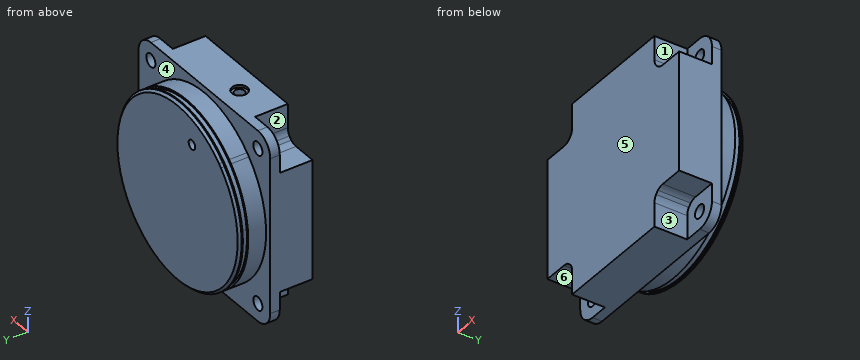
from build123d import *

# Parameters (mm, degrees)
F1_DEPTH        = 58
F0_R            = 5.5
F2_DEPTH        = 35.5
F3_DEPTH        = 35.5
F3_COPIES_COUNT = 4
F4_DEPTH        = 27.5
F4_COPIES_COUNT = 4
F5_SIZE         = 2
F7_D            = 8.5
F7_DEPTH        = 35
F7_CBORE_D      = 13
F7_CBORE_DEPTH  = 2
F7_TIP          = 2.5536576309
F9_D            = 8
F9_DEPTH        = 40
F9_TIP          = 2.4034424761
F10_W           = 4.5
F10_H           = 1.5


# Not quite as in the source:
# - a pattern or mirror of a feature is missing from the dataset's text; its kind, count and spacing are read off the source's solid


with BuildPart() as f1:
    # F0 (on Front) → F1 (new body)
    with BuildSketch(Plane.XZ):
        with BuildLine():
            ThreePointArc((-51.8845091547, 54.1571575119), (-52.9289321881, 52.9289321881), (-54.1571575119, 51.8845091547))
            ThreePointArc((-54.1571575119, 51.8845091547), (-27.9572279259, -69.5944926463), (75, 0))
            ThreePointArc((75, 0), (29.4419922338, 68.979483133), (-51.8845091547, 54.1571575119))
        make_face()
        with BuildLine():
            ThreePointArc((-51.8845091547, 54.1571575119), (-53.033008589, 53.033008589), (-54.1571575119, 51.8845091547))
            ThreePointArc((-54.1571575119, 51.8845091547), (-52.9289321881, 52.9289321881), (-51.8845091547, 54.1571575119))
        make_face()
    extrude(amount=-F1_DEPTH)

    # F0 (on Front) → F2 (join)
    with BuildSketch(Plane.XZ):
        with BuildLine():
            Line((-65, -80), (65, -80))
            ThreePointArc((65, -80), (75.6066017178, -75.6066017178), (80, -65))
            Line((80, -65), (80, 65))
            ThreePointArc((80, 65), (75.6066017178, 75.6066017178), (65, 80))
            Line((65, 80), (-50, 80))
            Line((-50, 80), (-50, 60))
            ThreePointArc((-50, 60), (-50.4827811717, 56.9303834484), (-51.8845091547, 54.1571575119))
            ThreePointArc((-51.8845091547, 54.1571575119), (29.4419922338, 68.979483133), (75, 0))
            ThreePointArc((75, 0), (-27.9572279259, -69.5944926463), (-54.1571575119, 51.8845091547))
            ThreePointArc((-54.1571575119, 51.8845091547), (-56.9303834484, 50.4827811717), (-60, 50))
            Line((-60, 50), (-80, 50))
            Line((-80, 50), (-80, -65))
            ThreePointArc((-80, -65), (-75.6066017178, -75.6066017178), (-65, -80))
        make_face()
        with BuildLine():
            Line((-80, 65), (-80, 50))
            Line((-80, 50), (-60, 50))
            ThreePointArc((-60, 50), (-56.9303834484, 50.4827811717), (-54.1571575119, 51.8845091547))
            ThreePointArc((-54.1571575119, 51.8845091547), (-53.033008589, 53.033008589), (-51.8845091547, 54.1571575119))
            ThreePointArc((-51.8845091547, 54.1571575119), (-50.4827811717, 56.9303834484), (-50, 60))
            Line((-50, 60), (-50, 80))
            Line((-50, 80), (-65, 80))
            ThreePointArc((-65, 80), (-75.6066017178, 75.6066017178), (-80, 65))
        make_face()
        with Locations((-65, 65)):
            Circle(F0_R, mode=Mode.SUBTRACT)
        with Locations((-65, 65)):
            Circle(F0_R)
    extrude(amount=-F2_DEPTH)

    # F0 (on Front) → F3 (cut, through all)
    with BuildSketch(Plane.XZ):
        with Locations((-65, 65)):
            Circle(F0_R)
    f3 = extrude(amount=-F3_DEPTH, mode=Mode.SUBTRACT)

    # F3_copies: F3 ×4 about axis
    f3_copies_axis = Axis((0, 0, 0), (0, 1, 0))
    for i in range(1, F3_COPIES_COUNT):
        add(f3.rotate(f3_copies_axis, i * 360 / F3_COPIES_COUNT), mode=Mode.SUBTRACT)

    # F0 (on Front) → F4 (cut)
    with BuildSketch(Plane.XZ):
        with BuildLine():
            Line((-80, 65), (-80, 50))
            Line((-80, 50), (-60, 50))
            ThreePointArc((-60, 50), (-56.9303834484, 50.4827811717), (-54.1571575119, 51.8845091547))
            ThreePointArc((-54.1571575119, 51.8845091547), (-53.033008589, 53.033008589), (-51.8845091547, 54.1571575119))
            ThreePointArc((-51.8845091547, 54.1571575119), (-50.4827811717, 56.9303834484), (-50, 60))
            Line((-50, 60), (-50, 80))
            Line((-50, 80), (-65, 80))
            ThreePointArc((-65, 80), (-75.6066017178, 75.6066017178), (-80, 65))
        make_face()
        with Locations((-65, 65)):
            Circle(F0_R, mode=Mode.SUBTRACT)
    f4 = extrude(amount=-F4_DEPTH, mode=Mode.SUBTRACT)

    # F4_copies: F4 ×4 about axis
    f4_copies_axis = Axis((0, 0, 0), (0, 1, 0))
    for i in range(1, F4_COPIES_COUNT):
        add(f4.rotate(f4_copies_axis, i * 360 / F4_COPIES_COUNT), mode=Mode.SUBTRACT)

    # F5
    f5_edges = [f1.edges().sort_by_distance(p)[0] for p in [
        (-75, 58, 0),
    ]]
    chamfer(f5_edges, length=F5_SIZE)

    # F7
    with Locations(Plane.XY.offset(80)):
        with Locations((-17.5, 18)):
            CounterBoreHole(F7_D / 2, F7_CBORE_D / 2, F7_CBORE_DEPTH, depth=F7_DEPTH)
            with Locations((0, 0, -(F7_DEPTH + F7_TIP / 2))):  # 118° drill point
                Cone(0, F7_D / 2, F7_TIP, mode=Mode.SUBTRACT)

    # F9
    with Locations(Plane(origin=(0, 58, 0), x_dir=(-1, 0, 0), z_dir=(0, 1, 0))):
        with Locations((17.5, 50)):
            Hole(F9_D / 2, depth=F9_DEPTH)
            with Locations((0, 0, -(F9_DEPTH + F9_TIP / 2))):  # 118° drill point
                Cone(0, F9_D / 2, F9_TIP, mode=Mode.SUBTRACT)

    # F10 (on Right) → F11 (revolve, cut)
    with BuildSketch(Plane.YZ):
        with Locations((52.75, 74.25)):
            Rectangle(F10_W, F10_H)
    revolve(axis=Axis((0, 29, 0), (0, 1, 0)), mode=Mode.SUBTRACT)


solid = f1.part
Read the model definition and answer for the solid it produces. Units are mm, in the model's axes. Face numbers are marked on the shaded views. A direction names the side the tool comes from. Round coordinates to 2 decimals unless told otherwise and drop trailing zeros. Write each loop counter-clockwise with the first axis right and the second up, starting at its lowest first coordinate (ties: lowest second). Pieces come first, ordered by that corner, then holes.
Q1. Find section C-C on y = 41.5. Determine the outline of the cut face in (x, z).
Values:
outline: circle Ø150 at (0, 0); hole circle Ø8 at (-17.5, 50)
Q2. A tool of negligible diameter and unlimited length cuts with its end or side. For the marked faces 1, 2 and 3, from which of +Z, -Z, +X, -X, +Y, -Y can it reach the whole face along a straight path? Write none if from no direction.
Values:
face 1: +Z, +X, -Y
face 2: +Z, -X, -Y
face 3: -Z, +X, -Y
Q3. Find section A-A on y = 7.5. Determine the outline of the cut face in (x, z).
Values:
outline: (-80, -50) - (-60, -50) arc R10 cw to (-54.16, -51.88) arc R75 ccw to (-51.88, -54.16) arc R10 cw to (-50, -60) - (-50, -80) - (50, -80) - (50, -60) arc R10 cw to (51.88, -54.16) arc R75 ccw to (54.16, -51.88) arc R10 cw to (60, -50) - (80, -50) - (80, 50) - (60, 50) arc R10 cw to (54.16, 51.88) arc R75 ccw to (51.88, 54.16) arc R10 cw to (50, 60) - (50, 80) - (-50, 80) - (-50, 60) arc R10 cw to (-51.88, 54.16) arc R75 ccw to (-54.16, 51.88) arc R10 cw to (-60, 50) - (-80, 50) - close
Q4. Flat-ended cylindrical pins translate along their axes: P1, Ø6.5, axis at x = -17.5, z = 50, coming from the +Y side; P2, Ø10, axis at x = 35.5, z = -47, coming from the -Y side; P3, Ø15, axis at x = 70, z = -60.5, coming from the -Y side; P4, Ø6, axis at x = -73, y = 19.5, coming from the -Z side. Find the tip coordinate at first contact, or state that the pin passes through.
Values:
P1: stops at y = 15.26
P2: stops at y = 0
P3: stops at y = 27.5
P4: stops at z = -50
Q5. Straight lines are drawn through the part: line 1 (Z direction, x = 65, y = 30); line 2 (X direction, y = 31, z = 50); line 3 (Y direction, x = 58, z = -71). For each, find the intervals that lie inside material, in ascending order.
Values:
line 1: z = -80 to -70.5, -59.5 to 59.5, 70.5 to 80
line 2: x = -80 to -21.5, -13.5 to 80
line 3: y = 27.5 to 35.5
Q6. The mould has two halves that part along Y. Classify the marked faces 4, 5 and 6: released by +Y, released by -Y, zero draft, split by the parting line, or undercut.
Values:
face 4: released by +Y
face 5: released by -Y
face 6: zero draft
Q7. Find section B-B on x = 0. Determine the outline of the cut face in (y, z), and give its area (3 significant figures).
Values:
outline: (0, -80) - (35.5, -80) - (35.5, -75) - (50.5, -75) - (50.5, -73.5) - (55, -73.5) - (55, -75) - (56, -75) - (58, -73) - (58, 73) - (56, 75) - (55, 75) - (55, 73.5) - (50.5, 73.5) - (50.5, 75) - (35.5, 75) - (35.5, 80) - (0, 80) - close
area: 9,040 mm2
